Job drawing, mm, ordinate dimensions from the low corner. One solid piece. Coordinates: 2 decimals unless noted, no trailing zeros. Order: outer loops, then holes, each group sorted by start corner. A loop starts at its lowest first (then second) coordinate and runs counter-clockwise, first axis right, second up. Notation, with made-up numbers: (24, -7.5) - (38, -7.5) arc R10 ccw to (38, 7.5) - close; hole circle Ø1 at (78.25, -9). An arc over 180 degrees is marked (long way). Use one line per item in the form item = value.
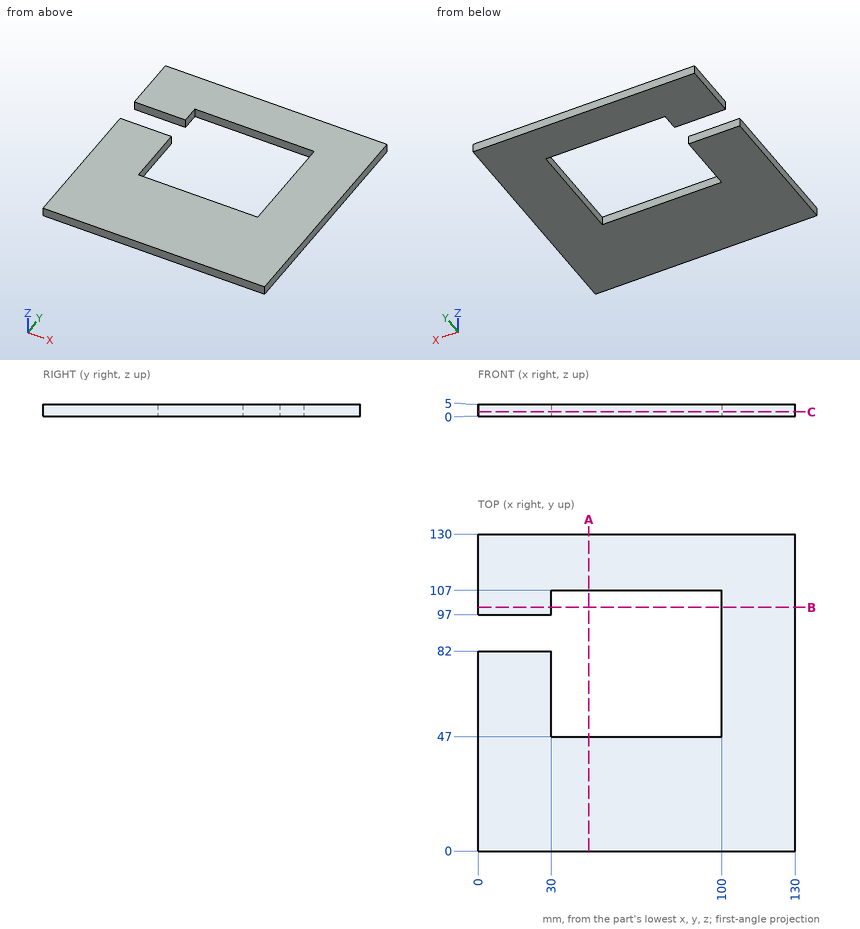
Item 1: Cut at C-C, the plane z = 1.75. Write the cut outline in (x, y), plus the area to 4 significant figures.
Derived:
outline = (0, 0) - (130, 0) - (130, 130) - (0, 130) - (0, 97) - (30, 97) - (30, 107) - (100, 107) - (100, 47) - (30, 47) - (30, 82) - (0, 82) - close
area = 12,250 mm²
Item 2: Cut at A-A, the plane x = 45.5. Write the cut outline in (y, z).
Derived:
outline = (0, 0) - (47, 0) - (47, 5) - (0, 5) - close; (107, 0) - (130, 0) - (130, 5) - (107, 5) - close
Item 3: Cut at B-B, the plane y = 100. Write the cut outline in (x, z), plus the area to 3 significant figures.
Derived:
outline = (0, 0) - (30, 0) - (30, 5) - (0, 5) - close; (100, 0) - (130, 0) - (130, 5) - (100, 5) - close
area = 300 mm²
Item 4: Drill centre lines: line 1 (X direction, y = 70, z = 2.25); line 2 (Y direction, x = 99, z = 0.4); line 3 (Y direction, x = 18, z = 3.25). Where is each one in solid material? Low to high. Write a range as [from, to].
Derived:
line_1 = [0, 30], [100, 130]
line_2 = [0, 47], [107, 130]
line_3 = [0, 82], [97, 130]
